Autodesk Inventor part; units mm, degrees
ref_plane "YZ Plane" through (0, 0, 0) normal (1, 0, 0) x (0, 1, 0)
ref_plane "XZ Plane" through (0, 0, 0) normal (0, 1, 0) x (-1, 0, 0)
ref_plane "XY Plane" through (0, 0, 0) normal (0, 0, 1) x (1, 0, 0)
sketch "Sketch1" plane through (0, 0, 0) normal (1, 0, 0) x (0, 1, 0)
  line L0 (0, 0) -> (8, 0)
  line L1 (8, 0) -> (8, 16)
  line L2 (8, 16) -> (0, 16)
  line L3 (0, 16) -> (0, 0)
  line L4 (8, 15) -> (2.5, 15)
  line L5 (8, 8) -> (2.5, 8)
  line L6 (6, 15) -> (6, 8)
  line L7 (2.5, 16) -> (2.5, 0)
  dimension "d7" = 8
  dimension "d8" = 16
  dimension "d9" = 1
  dimension "d10" = 7
  dimension "d11" = 6
  dimension "d12" = 2.5
revolve "Revolution1" add sketch "Sketch1" angle 360 about axis through (0, 0, 16) along (0, 0, 1) contours L7 L5 L1 L0 | L7 L4 L6 L5 | L2 L1 L4 L7
properties part number "belt_gear_1"
Here's how the part is built. I have some questions about the finished solid (model axes, mm). A direction names the side the tool comes from. Give positions to 0.01 mm unless a question says otherwise; leave off trailing zeros. Order: outer loops, then holes, each group sorted by start corner. A loop starts at its lowest first (then second) coordinate and runs counter-clockwise, first axis right, second up. Notation, with made-up numbers: (-24.75, 19.5) -> (3.25, 19.5) arc R15 cw to (3.25, 41.5) -> close; hole circle Ø2 at (0, 60.25). An arc over 180 degrees is marked (long way). Use a Markdown table: item, result. Add a question column.
Item 1: If we mould it in two halves opening along Y, with no side actions, what happens to faces 1 (the face through (0, -6, 11)), 2 (the face through (2, -2, 0)), 3 (the face through (-2.44, -0.54, 7.89))? For each: pulls with the +Y half, pulls with the -Y half, needs draft (parallel to the pull), parting line crosses it, or undercut.
Item 2: Imagine slicing it at C-C on z = 13. Please give me the cut outline in (x, y), plus the area to 3 significant figures.
Item 3: For faces 4 (the face through (-6, -2, 15)), 5 (the face through (7.81, -1.73, 15.51)), which set-ups out of +Z, -Z, +X, -X, +Y, -Y let a thin tool reach every point of the face, with its end or its side?
Item 4: Imagine slicing it at D-D on y = -3.25. Please give me the cut outline in (x, z), plus the area to 3 significant figures.
Item 5: I need wall thicknesses on line 1 (Z direction, x = -5.5, y = 4.5); line 2 (X direction, y = 0, z = 5); line 3 (Y direction, x = 0, z = 12). Which ranges of each line are inside material? Lowest first, please.
Item 6: Will these pins go through, and if not, where does the flat tip stop? pin 1 (2 mm diameter, centred on x = 6.5, z = 6, fed in from +Y); pin 2 (5 mm diameter, centred on x = 5, z = 11, fed in from -Y).
Item 7: Imagine slicing it at A-A on x = 0. Please give me the cut outline in (y, z), plus the area to 3 significant figures.
Data:
| question | item | result |
|---|---|---|
| 1 | face 1 | parting line crosses it |
| 1 | face 2 | needs draft |
| 1 | face 3 | undercut |
| 2 | outline | circle Ø12 at (0, 0); hole circle Ø5 at (0, 0) |
| 2 | area | 93.5 mm² |
| 3 | face 4 | none |
| 3 | face 5 | +Z, -Z |
| 4 | outline | (-7.31, 0) -> (7.31, 0) -> (7.31, 8) -> (5.04, 8) -> (5.04, 15) -> (7.31, 15) -> (7.31, 16) -> (-7.31, 16) -> (-7.31, 15) -> (-5.04, 15) -> (-5.04, 8) -> (-7.31, 8) -> close |
| 4 | area | 202 mm² |
| 5 | line 1 | z = 0 to 8, 15 to 16 |
| 5 | line 2 | x = -8 to -2.5, 2.5 to 8 |
| 5 | line 3 | y = -6 to -2.5, 2.5 to 6 |
| 6 | pin 1 | stops at y = 5.81 |
| 6 | pin 2 | stops at y = -5.45 |
| 7 | outline | (-8, 0) -> (-2.5, 0) -> (-2.5, 16) -> (-8, 16) -> (-8, 15) -> (-6, 15) -> (-6, 8) -> (-8, 8) -> close; (2.5, 0) -> (8, 0) -> (8, 8) -> (6, 8) -> (6, 15) -> (8, 15) -> (8, 16) -> (2.5, 16) -> close |
| 7 | area | 148 mm² |
